Input: part model. Units: mm. Frame: model coordinates. Round coordinates to 2 decimals unless told otherwise and drop trailing zeros. Write each loop counter-clockwise with the first axis right and the second up, starting at its lowest first coordinate (ties: lowest second). Pieces come first, ordered by that corner, then holes. Notation, with made-up numbers: (41, 4) - (68, 4) arc R22 cw to (68, 16) - close; hole circle Ø6 at (21.5, 17.25). An arc over 180 degrees is marked (long way). Use one line per item in the form item = value.
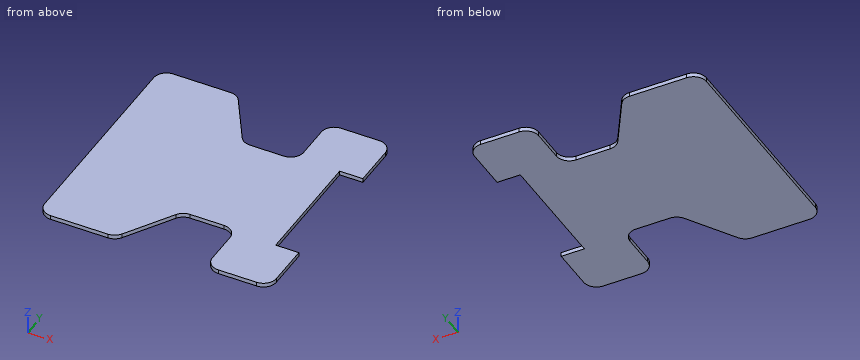
```python
from build123d import *

# Parameters (mm, degrees)
BOSS_EXTRUDE1_DEPTH = 1.6
SKETCH2_OUTSIDE_W   = 117.458
SKETCH2_OUTSIDE_H   = 117.458
CUT_EXTRUDE1_DEPTH  = 128.289276846
FILLET2_R           = 5


with BuildPart() as part:
    # Sketch1 → Boss-Extrude1 (new body)
    with BuildSketch(Plane.XY):
        Polygon((90, 68.5), (90, 90), (0, 90), (0, 0), (90, 0), (90, 21.5), (81, 21.5), (81, 68.5), align=None)
    extrude(amount=BOSS_EXTRUDE1_DEPTH)

    # Sketch2 outside → Cut-Extrude1 (cut, through all)
    with BuildSketch(Plane.XY.offset(1.6)):
        with Locations((45, 45)):
            Rectangle(SKETCH2_OUTSIDE_W, SKETCH2_OUTSIDE_H)
        Polygon((0, 90), (30, 90), (44.142135624, 67), (65.142135624, 67), (65.142135624, 90), (90, 90), (90, 68.5), (81, 68.5), (81, 21.5), (90, 21.5), (90, 0), (65.142135624, 0), (65.142135624, 23), (44.142135624, 23), (30, 0), (0, 0), align=None, mode=Mode.SUBTRACT)
    extrude(amount=-CUT_EXTRUDE1_DEPTH, mode=Mode.SUBTRACT)

    # Fillet2
    fillet2_edges = [part.edges().sort_by_distance(p)[0] for p in [
        (0, 90, 0.8),
        (90, 90, 0.8),
        (90, 0, 0.8),
        (0, 0, 0.8),
        (30, 90, 0.8),
        (44.142135624, 67, 0.8),
        (65.142135624, 67, 0.8),
        (65.142135624, 90, 0.8),
        (65.142135624, 0, 0.8),
        (65.142135624, 23, 0.8),
        (44.142135624, 23, 0.8),
        (30, 0, 0.8),
    ]]
    fillet(fillet2_edges, radius=FILLET2_R)


solid = part.part
```
(1) Cut plane A-A on y = 16.5. Output: boundary loops of the cut face in (x, z).
Derived:
outline = (0, 0) - (40.15, 0) - (40.15, 1.6) - (0, 1.6) - close; (65.14, 0) - (90, 0) - (90, 1.6) - (65.14, 1.6) - close
(2) Cut plane D-D on y = 53.5. Output: boundary loops of the cut face in (x, z), then the cut area to 3 significant figures.
Derived:
outline = (0, 0) - (81, 0) - (81, 1.6) - (0, 1.6) - close
area = 130 mm^2
(3) Cut plane B-B on z = 0.9. Output: boundary loops of the cut face in (x, y).
Derived:
outline = (0, 5) arc R5 ccw to (5, 0) - (27.2, 0) arc R5 ccw to (31.46, 2.38) - (42.68, 20.62) arc R5 cw to (46.94, 23) - (60.14, 23) arc R5 cw to (65.14, 18) - (65.14, 5) arc R5 ccw to (70.14, 0) - (85, 0) arc R5 ccw to (90, 5) - (90, 21.5) - (81, 21.5) - (81, 68.5) - (90, 68.5) - (90, 85) arc R5 ccw to (85, 90) - (70.14, 90) arc R5 ccw to (65.14, 85) - (65.14, 72) arc R5 cw to (60.14, 67) - (46.94, 67) arc R5 cw to (42.68, 69.38) - (31.46, 87.62) arc R5 ccw to (27.2, 90) - (5, 90) arc R5 ccw to (0, 85) - close
(4) First-contact query: pin 1 Ø0.8 at (y, z) = (33.5, 0.5) entering from +X; pin 2 Ø0.8 at (x, z) = (87.5, 0.5) entering from +Y. Flat tips, straight axial feed; report the tip coordinate or a pass-through.
Derived:
pin_1 = 81
pin_2 = 89.54
(5) Material intervals for L1, parallel to Y at x = 82.5, z = 1; L2, parallel to Y at x = 52, z = 1.2; L3, parallel to X at y = 43.5, z = 0.95, sorted ascending.
Derived:
L1 = 0 to 21.5, 68.5 to 90
L2 = 23 to 67
L3 = 0 to 81
(6) Cut plane C-C on x = 49. Output: boundary loops of the cut face in (y, z).
Derived:
outline = (23, 0) - (67, 0) - (67, 1.6) - (23, 1.6) - close
